For this review, take the finished solid that the model builds, in its own axes (mm). Coordinates: 2 decimals unless noted, no trailing zeros. Write each loop counter-clockwise with the first axis right and the second up, starting at its lowest first coordinate (ties: lowest second). Pieces come first, ordered by that corner, then holes. Notation, with made-up numbers: M 40,1 L 45,1 A14 cw 45,27 Z; hole C -23,47 d6. An arc over 180 degrees is marked long. Return JSON: item names as keys, results as strings.
```python
from build123d import *

# Parameters (mm, degrees)
SKETCH1_W           = 10.166490401
SKETCH1_H           = 88.9
BOSS_EXTRUDE1_DEPTH = 10.16
CUT_LOFT1_DEPTH     = 9.5
SKETCH6_R           = 26.581471798
CUT_EXTRUDE2_DEPTH  = 12


# Read off the part's stored shape, not the designer's step: Cut-Loft1
with BuildPart() as part:
    # Sketch1 → Boss-Extrude1 (new body)
    with BuildSketch(Plane.XY):
        Polygon((-245, 2053.071580455), (-245, 2042.911580455), (-321.2, 2042.911580455), (-321.2, 2053.071580455), (-413.472915973, 2053.071580455), (-352.180527886, 0), (-270.8, 0), (-270.8, 10.16), (-220, 10.16), (-220, 0), (-55.8292, 0), (-55.8292, 10.16), (55.8292, 10.16), (55.8292, 0), (220, 0), (220, 10.16), (270.8, 10.16), (270.8, 0), (352.180527886, 0), (413.472915973, 2053.071580455), (321.2, 2053.071580455), (321.2, 2042.911580455), (245, 2042.911580455), (245, 2053.071580455), (38.1, 2053.071580455), (38.1, 2042.911580455), (-38.1, 2042.911580455), (-38.1, 2053.071580455), align=None)
        with Locations((-211.45202358, 1909.561580455)):
            Rectangle(SKETCH1_W, SKETCH1_H, mode=Mode.SUBTRACT)
        with Locations((-211.45202358, 1731.761580455)):
            Rectangle(SKETCH1_W, SKETCH1_H, mode=Mode.SUBTRACT)
        Polygon((-298.801924037, 122.832814726), (-292.291252627, 216.569681682), (-302.408932711, 217.272424291), (-308.919604121, 123.535557335), align=None, mode=Mode.SUBTRACT)
        Polygon((-286.484012658, 300.178951146), (-279.971498388, 393.942350533), (-290.089178472, 394.645093142), (-296.601692742, 300.881693756), align=None, mode=Mode.SUBTRACT)
        Polygon((-274.16610128, 477.525087567), (-267.651744149, 571.315019385), (-277.769424233, 572.017761994), (-284.283781364, 478.227830176), align=None, mode=Mode.SUBTRACT)
        Polygon((-261.848189901, 654.871223988), (-255.33198991, 748.687688236), (-265.449669994, 749.390430845), (-271.965869985, 655.573966597), align=None, mode=Mode.SUBTRACT)
        Polygon((-249.530278522, 832.217360408), (-243.012235672, 926.060357088), (-253.129915756, 926.763099697), (-259.647958606, 832.920103017), align=None, mode=Mode.SUBTRACT)
        Polygon((-237.212367144, 1009.563496829), (-230.692481433, 1103.433025939), (-240.810161517, 1104.135768548), (-247.330047228, 1010.266239438), align=None, mode=Mode.SUBTRACT)
        Polygon((-224.894455765, 1186.909633249), (-218.372727194, 1280.805694791), (-228.490407278, 1281.5084374), (-235.012135849, 1187.612375858), align=None, mode=Mode.SUBTRACT)
        Polygon((-206.36877838, 1453.631580489), (-216.535268781, 1453.631580489), (-222.69422447, 1364.958512279), (-212.576544386, 1364.25576967), align=None, mode=Mode.SUBTRACT)
        Polygon((216.535268781, 1453.631580489), (206.36877838, 1453.631580489), (212.576544386, 1364.25576967), (222.69422447, 1364.958512279), align=None, mode=Mode.SUBTRACT)
        Polygon((218.372727194, 1280.805694791), (224.894455765, 1186.909633249), (235.012135849, 1187.612375858), (228.490407278, 1281.5084374), align=None, mode=Mode.SUBTRACT)
        Polygon((230.692481433, 1103.433025939), (237.212367144, 1009.563496829), (247.330047228, 1010.266239438), (240.810161517, 1104.135768548), align=None, mode=Mode.SUBTRACT)
        Polygon((243.012235672, 926.060357088), (249.530278522, 832.217360408), (259.647958606, 832.920103017), (253.129915756, 926.763099697), align=None, mode=Mode.SUBTRACT)
        Polygon((255.33198991, 748.687688236), (261.848189901, 654.871223988), (271.965869985, 655.573966597), (265.449669994, 749.390430845), align=None, mode=Mode.SUBTRACT)
        Polygon((267.651744149, 571.315019385), (274.16610128, 477.525087567), (284.283781364, 478.227830176), (277.769424233, 572.017761994), align=None, mode=Mode.SUBTRACT)
        Polygon((279.971498388, 393.942350533), (286.484012658, 300.178951146), (296.601692742, 300.881693756), (290.089178472, 394.645093142), align=None, mode=Mode.SUBTRACT)
        Polygon((292.291252627, 216.569681682), (298.801924037, 122.832814726), (308.919604121, 123.535557335), (302.408932711, 217.272424291), align=None, mode=Mode.SUBTRACT)
        with Locations((211.45202358, 1731.761580455)):
            Rectangle(SKETCH1_W, SKETCH1_H, mode=Mode.SUBTRACT)
        with Locations((-211.45202358, 1553.961580455)):
            Rectangle(SKETCH1_W, SKETCH1_H, mode=Mode.SUBTRACT)
        with Locations((211.45202358, 1553.961580455)):
            Rectangle(SKETCH1_W, SKETCH1_H, mode=Mode.SUBTRACT)
        with Locations((211.45202358, 1909.561580455)):
            Rectangle(SKETCH1_W, SKETCH1_H, mode=Mode.SUBTRACT)
    extrude(amount=BOSS_EXTRUDE1_DEPTH)

    # Cut-Loft1 outline → Cut-Loft1 (cut)
    with BuildSketch(Plane.XY):
        Polygon((413.472915973, 2053.071580455), (380.911770747, 2053.071580455), (319.430777619, 0), (352.180527886, 0), align=None)
    cut_loft1 = extrude(amount=CUT_LOFT1_DEPTH, mode=Mode.SUBTRACT)

    # Mirror1: Cut-Loft1 across plane
    add(cut_loft1.mirror(Plane(origin=(0, 0, 0), x_dir=(0, 0, 1), z_dir=(1, 0, 0))), mode=Mode.SUBTRACT)

    # Sketch6 → Cut-Extrude2 (cut)
    with BuildSketch(Plane.XY.offset(10.16)):
        with Locations((28.844157405, 1657.225539641)):
            Circle(SKETCH6_R)
    extrude(amount=-CUT_EXTRUDE2_DEPTH, mode=Mode.SUBTRACT)


solid = part.part
```
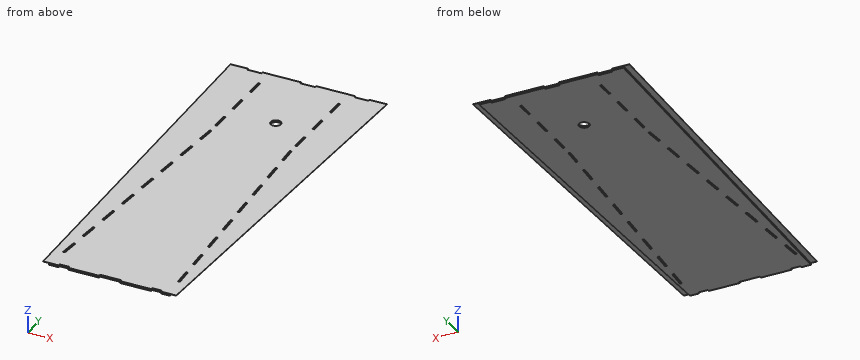
1. Clearance check with flat-ended pins moving along their axes: pin 1 Ø3 at (x, z) = (-284, 4) entering from +Y; pin 2 Ø5 at (x, y) = (-91.5, 253) entering from -Z; pin 3 Ø3 at (y, z) = (1896.5, 4.5) entering from +X; pin 4 Ø5 at (y, z) = (1587.5, 4.5) entering from +X. State where each tip first meets the part, or that it passes through.
Checks:
{"pin 1": "y = 2042.91", "pin 2": "z = 0", "pin 3": "x = 376.27", "pin 4": "x = 367.04"}
2. We need section C-C (z = 7). Give the number of separate pieces and of enclosed holes in the cut face, plus the area to 3 significant figures.
Checks:
{"separate pieces": "1", "enclosed holes": "23", "area": "1,410,000 mm2"}
3. We need section A-A (y = 701). State the section outline as (x, z) points.
Checks:
{"outline": "M -373.11,9.5 L -340.42,9.5 L -340.42,0 L -268.81,0 L -268.81,10.16 L -373.11,10.16 Z; M -258.64,0 L 258.64,0 L 258.64,10.16 L -258.64,10.16 Z; M 268.81,0 L 340.42,0 L 340.42,9.5 L 373.11,9.5 L 373.11,10.16 L 268.81,10.16 Z"}
4. We need section B-B (y = 426). State the section outline as (x, z) points, plus the area to 3 significant figures.
Checks:
{"outline": "M -364.9,9.5 L -332.19,9.5 L -332.19,0 L 332.19,0 L 332.19,9.5 L 364.9,9.5 L 364.9,10.16 L -364.9,10.16 Z", "area": "6,790 mm2"}
5. Wall thickness on L1, parallel to X at y = 666, z = 4.5; L2, parallel to X at y = 492.5, z = 5.5; L3, parallel to Y at x = -287, z = 9.5: over which ranges is each line inside the solid? List them lowest first. Write a range as from..to.
Checks:
{"L1": "-339.37..-271.24, -261.08..261.08, 271.24..339.37", "L2": "-334.18..-283.29, -273.13..273.13, 283.29..334.18", "L3": "0..300.21, 394.43..2042.91"}
